Read the model definition and answer for the solid it produces. Units are mm, in the model's axes. Face numbers are marked on the shaded views. Give positions to 0.01 mm unless a question says otherwise; leave off trailing zeros. Order: outer loops, then holes, each group sorted by start corner. A loop starts at its lowest first (then second) coordinate and runs counter-clockwise, first axis right, second up.
Item 1: Find the intervals of material crossed by line 1 along Y through (x, z) = (0, -8); line 2 along Y through (x, z) = (12, -31.5); line 3 along X through (y, z) = (1, -16), in increasing order.
Item 2: A cutting plane is placed at A-A (z = -13). Write down the section's boundary in (x, y).
Item 3: The mould has two halves that part along X. Classify the marked faces 1, 2 and 3: +X half, -X half, draft (parallel to the pull), parting line (faces both ways), or undercut.
Item 4: Given pin 1 Ø5 at (x, z) = (16, -7.5) entering from -Y; pin 2 Ø4 at (x, z) = (30.5, -13.5) entering from +Y; pin 3 Ø1.5 at (y, z) = (30, -23) entering from +X, each flat-ended and moving along its own axis, determine where each tip first touches the part or whether it passes through.
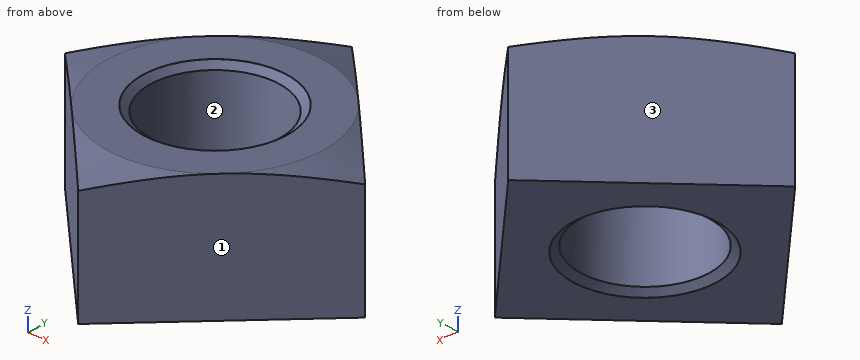
from build123d import *

# Parameters (mm, degrees)
BASENUT_START = -33.3502
BASENUTSKE_R  = 17.06626
BASENUT_DEPTH = 33.3502


with BuildPart() as part:
    # BaseNutSke → BaseNut (new body)
    with BuildSketch(Plane.XY.offset(BASENUT_START)):
        Polygon((40.411152545, 0), (0, 40.411152545), (-40.411152545, 0), (0, -40.411152545), align=None)
        Circle(BASENUTSKE_R, mode=Mode.SUBTRACT)
    extrude(amount=BASENUT_DEPTH)

    # EndChamferSketch → EndChamfer (revolve, cut)
    with BuildSketch(Plane(origin=(0, 0, 0), x_dir=(0, 0, -1), z_dir=(1, 0, 0)), mode=Mode.PRIVATE) as endchamfer_sk:
        Polygon((33.3248, 19.05), (31.797434837, 16.867886), (33.3502, 16.867886), (33.3502, 19.05), align=None)
        Polygon((0, 19.05), (0.0254, 19.05), (1.552765163, 16.867886), (0, 16.867886), align=None)
    revolve(endchamfer_sk.sketch.rotate(Axis((0, 0, -25.037505729), (0, 0, -1)), 90), axis=Axis((0, 0, -25.037505729), (0, 0, -1)), mode=Mode.SUBTRACT)

    # Sketch2 → Single-Chamfer (revolve, cut)
    with BuildSketch(Plane(origin=(0, 0, 0), x_dir=(0, 0, -1), z_dir=(1, 0, 0))):
        Polygon((-12.7, 28.575), (0, 28.575), (6.57444226, 53.111152545), (-12.7, 53.111152545), align=None)
    revolve(axis=Axis((0, 0, 0), (0, 0, -1)), mode=Mode.SUBTRACT)


solid = part.part
Response values:
1. line 1: y = -40.41 to -17.07, 17.07 to 40.41
1. line 2: y = -28.41 to -12.13, 12.13 to 28.41
1. line 3: x = -39.41 to -17.04, 17.04 to 39.41
2. outline: (-40.41, 0) - (0, -40.41) - (40.41, 0) - (0, 40.41) - close; hole circle Ø34.13 at (0, 0)
3. face 1: +X half
3. face 2: undercut
3. face 3: -X half
4. pin 1: stops at y = -26.91
4. pin 2: stops at y = 11.91
4. pin 3: stops at x = 11.16
